```python
from build123d import *

# Parameters (mm, degrees)
F4_SIZE = 1


# Not quite as in the source:
# - a fillet or chamfer that OpenCascade refuses, or shapes differently, is made with other operations: its cross-section is extruded or revolved along the edge and cut away or added


with BuildPart() as f1:
    # F0 (on Front) → F1 (revolve)
    with BuildSketch(Plane.XZ):
        with BuildLine():
            Line((0, 28), (0, 35))
            ThreePointArc((0, 35), (-17.3691143388, 19.6363209229), (-4.2406859855, 0.5215848098))
            Line((-4.2406859855, 0.5215848098), (-3.75, 28))
            Line((-3.75, 28), (0, 28))
        make_face()
    revolve(axis=Axis((0, 0, 16.7157072574), (0, 0, -1)))

    # F2: chamfer of 0.5 x 3 on 1 edges, made by hand

    # F2_s1 → F2_t2 (revolve, cut)
    with BuildSketch(Plane.XZ):
        with BuildLine():
            Line((-4.1607847025, 3.6471133949), (-4.8506659959, 0.5610496404))
            Line((-4.8506659959, 0.5610496404), (-4.8672070924, 0.5033747574))
            ThreePointArc((-4.8672070924, 0.5033747574), (-4.5463653864, 0.5387452771), (-4.2552254803, 0.4633731005))
            Line((-4.2552254803, 0.4633731005), (-4.1806955496, 0.520513552))
            ThreePointArc((-4.1806955496, 0.520513552), (-4.152785205, 2.0834928499), (-4.1007942666, 3.6460421371))
            Line((-4.1007942666, 3.6460421371), (-4.1607847025, 3.6471133949))
        make_face()
    revolve(axis=Axis((0, 0, 0.5215848098), (0, 0, -1)), mode=Mode.SUBTRACT)

    # F4
    f4_edges = [f1.edges().sort_by_distance(p)[0] for p in [
        (3.75, 0, 28),
    ]]
    chamfer(f4_edges, length=F4_SIZE)


solid = f1.part
```
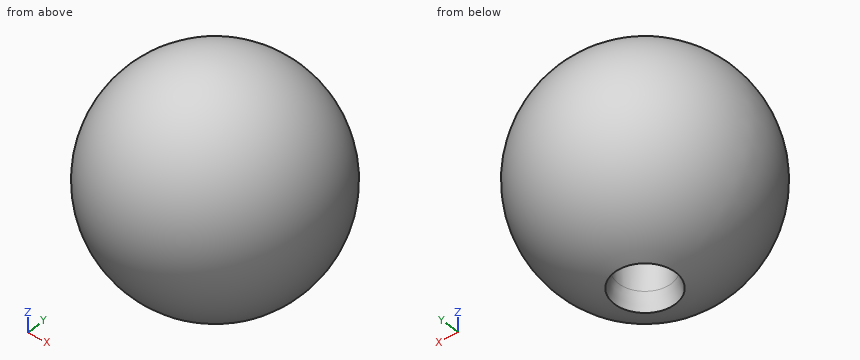
Source: CAD feature listing. Evaluate the final solid. Frame: model axes, mm. Round coordinates to 2 decimals unless told otherwise and drop trailing zeros. Order: outer loops, then holes, each group sorted by start corner. A loop starts at its lowest first (then second) coordinate and runs counter-clockwise, first axis right, second up. Notation, with made-up numbers: (16.25, 50.25) -> (71.25, 50.25) arc R26 ccw to (71.25, 81.25) -> close; hole circle Ø2 at (-21.75, -32). An arc over 180 degrees is marked (long way). Use CSV: the item, a comma, the result in double quotes.
(1) First-contact query: pin 1 Ø8 at (x, y) = (-4.5, -5) entering from +Z; pin 2 Ø1 at (y, z) = (7.5, 18.5) entering from -X; pin 3 Ø3 at (x, y) = (-2, 7) entering from +Z. Flat tips, straight axial feed; report the tip coordinate or a pass-through.
Report:
pin 1,"z = 34.79"
pin 2,"x = -16.01"
pin 3,"z = 34.02"
(2) Section C-C on z = 24. Return the cut outline in (x, y).
Report:
outline,"circle Ø32.5 at (0, 0); hole circle Ø7.64 at (0, 0)"
(3) Section B-B on y = 10.5. Return the cut outline in (x, z), and give its area (3 significant figures).
Report:
outline,"circle Ø28 at (0, 17.5)"
area,"616 mm^2"
(4) Section D-D on z = 17. Return the cut outline in (x, y), and give its area (3 significant figures).
Report:
outline,"circle Ø34.99 at (0, 0); hole circle Ø7.89 at (0, 0)"
area,"912 mm^2"
(5) Section A-A on z = 31.5. Return the cut outline in (x, y), and give its area (3 significant figures).
Report:
outline,"circle Ø21 at (0, 0)"
area,"346 mm^2"
(6) Ray query, L1, parallel to Y at x = 0, z = 13; L2, parallel to Z at x = 13, y = 6.5; L3, parallel to Y at x = 10, z = 10.5. Return the intervals inside material, ascending.
Report:
L1,"-16.91 to -4.02, 4.02 to 16.91"
L2,"7.75 to 27.25"
L3,"-12.54 to 12.54"
